Build history of the part. All positions in model axes, mm. Face numbers are marked on the shaded views. A direction names the side the tool comes from. Round coordinates to 2 decimals unless told otherwise and drop trailing zeros. Order: outer loops, then holes, each group sorted by start corner. A loop starts at its lowest first (then second) coordinate and runs counter-clockwise, first axis right, second up. Notation, with made-up numbers: M 16,39 L 61,39 A15 ccw 61,59 Z; hole C 4.5,52 d5. An arc over 180 degrees is marked long. One line per item, written item: value. Start each with the question number.
Item 1: Band-saw the part on A-A, the plane z = 7. Write the cut outline in (x, y).
Item 2: Probe L1, parallel to Z at x = 12.3, y = 0 (3 decimals); L2, parallel to Z at x = 14.55, y = 0; L3, parallel to X at y = -8, z = 7. List the from-to ranges inside material, lowest first.
Item 3: Tool access for the marked faces 1 and 2: list every direction of +Z, -Z, +X, -X, +Y, -Y with a clear straight run to the whole face (end or side of a thin tool).
Item 4: Band-saw the part on D-D, the plane x = 8.5. Write the cut outline in (y, z).
Item 5: Band-saw the part on B-B, the plane z = 17.75. Write the cut outline in (x, y) (3 decimals), then the cut area to 3 significant figures.
Item 6: Pin check, flat tips, straight feed: pin 1 (2.5 mm diameter, centred on y = -1.5, z = 17, fed in from +X); pin 2 (1 mm diameter, centred on x = -15, y = 10, fed in from -Z); pin 3 (4 mm diameter, centred on x = -7, z = 21, fed in from +Y). Stop position of each tip, or through.
Item 7: Two-plate mould, pull along X, no slides. Class the marked faces 3, 4 and 5: +X half, -X half, draft (parallel to the pull), parting line (faces both ways), or undercut.
```python
from build123d import *

# Parameters (mm, degrees)
SKETCH1_W               = 32
SKETCH1_H               = 27
BOSS_EXTRUDE1_DEPTH     = 35
FILLET1_R               = 2
CUT_EXTRUDE1_DEPTH      = 1
CUT_EXTRUDE1_DEPTH_BACK = 28
BOSS_EXTRUDE2_DEPTH     = 7
BOSS_EXTRUDE3_DEPTH     = 1.75
SKETCH5_W               = 2
SKETCH5_H               = 7
CUT_EXTRUDE2_DEPTH      = 33
CUT_EXTRUDE3_DEPTH      = 20
SKETCH7_W               = 2
SKETCH7_H               = 33
BOSS_EXTRUDE4_DEPTH     = 0.25
FILLET2_R               = 6
CUT_EXTRUDE5_DEPTH      = 4.5
SKETCH14_W              = 2.5
SKETCH14_H              = 20
CUT_EXTRUDE6_DEPTH      = 20
SKETCH16_W              = 2
SKETCH16_H              = 3.75
SKETCH16_H_2            = 2
BOSS_EXTRUDE5_DEPTH     = 20
BOSS_EXTRUDE6_DEPTH     = 20


with BuildPart() as part:
    # Sketch1 → Boss-Extrude1 (new body)
    with BuildSketch(Plane.XY):
        Rectangle(SKETCH1_W, SKETCH1_H)
    extrude(amount=BOSS_EXTRUDE1_DEPTH)

    # Fillet1
    fillet1_edges = [part.edges().sort_by_distance(p)[0] for p in [
        (16, -13.5, 17.5),
        (-16, -13.5, 17.5),
        (-16, 13.5, 17.5),
        (16, 13.5, 17.5),
    ]]
    fillet(fillet1_edges, radius=FILLET1_R)

    # Sketch2 → Cut-Extrude1 (cut, two sides)
    with BuildSketch(Plane.XZ.offset(13.5)) as cut_extrude1_sk:
        Polygon((-7.75, 0), (-7.75, 1.75), (-9.25, 1.75), (-9.25, 5.25), (9.25, 5.25), (9.25, 1.75), (7.75, 1.75), (7.75, 0), align=None)
    extrude(amount=CUT_EXTRUDE1_DEPTH, mode=Mode.SUBTRACT)
    extrude(cut_extrude1_sk.sketch, amount=-CUT_EXTRUDE1_DEPTH_BACK, mode=Mode.SUBTRACT)

    # Sketch3 → Boss-Extrude2 (add)
    with BuildSketch(Plane.XZ.offset(13.5)):
        Polygon((-7.75, 0), (-7.75, 1.75), (-9.25, 1.75), (-9.25, 5.25), (9.25, 5.25), (9.25, 1.75), (7.75, 1.75), (7.75, 0), align=None)
    extrude(amount=-BOSS_EXTRUDE2_DEPTH)

    # Sketch4 → Boss-Extrude3 (add)
    with BuildSketch(Plane(origin=(0, 0, 1.75), x_dir=(-1, 0, 0), z_dir=(0, 0, -1))):
        with BuildLine():
            Line((-7.75, 6.5), (-7.75, 5.5))
            ThreePointArc((-7.75, 5.5), (-7.5, 6), (-7.75, 6.5))
        make_face()
    boss_extrude3 = extrude(amount=BOSS_EXTRUDE3_DEPTH)

    # Mirror1: Boss-Extrude3 across plane
    add(boss_extrude3.mirror(Plane(origin=(0, 0, 0), x_dir=(0, 0, 1), z_dir=(1, 0, 0))))

    # Sketch5 → Cut-Extrude2 (cut)
    with BuildSketch(Plane(origin=(0, 0, 0), x_dir=(-1, 0, 0), z_dir=(0, 0, -1))):
        with Locations((0, -10)):
            Rectangle(SKETCH5_W, SKETCH5_H)
    extrude(amount=-CUT_EXTRUDE2_DEPTH, mode=Mode.SUBTRACT)

    # Sketch6 → Cut-Extrude3 (cut)
    with BuildSketch(Plane(origin=(0, 13.5, 0), x_dir=(1, 0, 0), z_dir=(0, 1, 0))):
        Polygon((-12.5, -7.75), (-12.5, -9.25), (-11.5, -9.25), (-11.5, -33), (11.5, -33), (11.5, -9.25), (12.5, -9.25), (12.5, -7.75), align=None)
    extrude(amount=-CUT_EXTRUDE3_DEPTH, mode=Mode.SUBTRACT)

    # Sketch7 → Boss-Extrude4 (add)
    with BuildSketch(Plane.XZ.offset(13.5)):
        with Locations((0, 16.5)):
            Rectangle(SKETCH7_W, SKETCH7_H)
    extrude(amount=-BOSS_EXTRUDE4_DEPTH)

    # Fillet2
    fillet2_edges = [part.edges().sort_by_distance(p)[0] for p in [
        (0, -13.25, 33),
    ]]
    fillet(fillet2_edges, radius=FILLET2_R)

    # Sketch9 → Cut-Revolve1 (revolve, cut)
    with BuildSketch(Plane(origin=(0, 0, 17.75), x_dir=(-1, 0, 0), z_dir=(0, 0, -1))):
        Polygon((-15, 4.25), (-14, 4.25), (-14, 3.325), (-11.5, 3.325), (-11.5, 0), (-16, 0), (-16, 3.75), (-15, 3.75), align=None)
    revolve(axis=Axis((16, 0, 17.75), (-1, 0, 0)), mode=Mode.SUBTRACT)

    # Sketch11 → Cut-Extrude5 (cut)
    with BuildSketch(Plane(origin=(-16, 0, 44), x_dir=(0, 0, -1), z_dir=(1, 0, 0))):
        with BuildLine():
            Line((24.25, 23), (24.25, 0))
            ThreePointArc((24.25, 0), (21, -3.25), (17.75, 0))
            Line((17.75, 0), (17.75, 23))
            ThreePointArc((17.75, 23), (21, 26.25), (24.25, 23))
        make_face()
    extrude(amount=CUT_EXTRUDE5_DEPTH, mode=Mode.SUBTRACT)

    # Sketch14 → Cut-Extrude6 (cut)
    with BuildSketch(Plane(origin=(0, 13.5, 0), x_dir=(1, 0, 0), z_dir=(0, 1, 0))):
        with Locations((-12.75, -23)):
            Rectangle(SKETCH14_W, SKETCH14_H)
    extrude(amount=-CUT_EXTRUDE6_DEPTH, mode=Mode.SUBTRACT)

    # Sketch16 → Boss-Extrude5 (add)
    with BuildSketch(Plane(origin=(0, 13.5, 0), x_dir=(1, 0, 0), z_dir=(0, 1, 0))):
        with Locations((-11, -13.125)):
            Rectangle(SKETCH16_W, SKETCH16_H)
        with Locations((-11, -32)):
            Rectangle(SKETCH16_W, SKETCH16_H_2)
    extrude(amount=-BOSS_EXTRUDE5_DEPTH)

    # Sketch20 → Boss-Extrude6 (add)
    with BuildSketch(Plane(origin=(0, 13.5, 0), x_dir=(1, 0, 0), z_dir=(0, 1, 0))):
        Polygon((-11.5, -9.25), (-10, -11.25), (-11.5, -11.25), align=None)
        Polygon((-10, -31), (-8.5, -33), (-10, -33), align=None)
    extrude(amount=-BOSS_EXTRUDE6_DEPTH)


solid = part.part
```
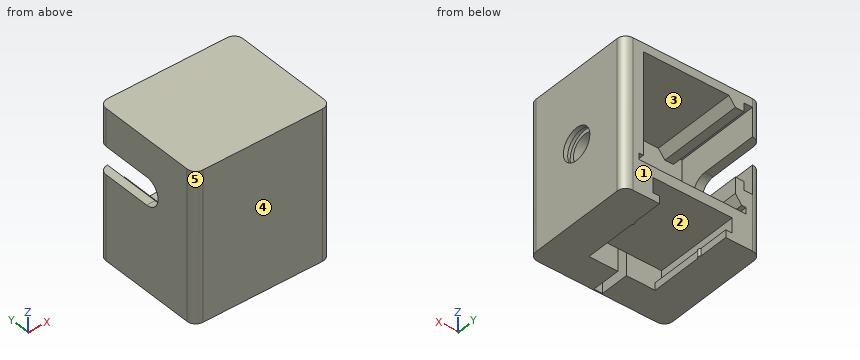
Output:
1. outline: M -16,-11.5 A2 ccw -14,-13.5 L 14,-13.5 A2 ccw 16,-11.5 L 16,11.5 A2 ccw 14,13.5 L -14,13.5 A2 ccw -16,11.5 Z; hole M -1,-13.25 L 1,-13.25 L 1,-6.5 L -1,-6.5 Z
2. L1: z = 0 to 7.75, 9.25 to 14.425, 21.075 to 35
2. L2: z = 0 to 13.5, 22 to 35
2. L3: x = -16 to -1, 1 to 16
3. face 1: +Z, -Z, +X, -X, +Y
3. face 2: +Y
4. outline: M -13.5,0 L 13.5,0 L 13.5,1.75 L -6.5,1.75 L -6.5,5.25 L 13.5,5.25 L 13.5,7.75 L -6.5,7.75 L -6.5,33 L 13.5,33 L 13.5,35 L -13.5,35 Z
5. outline: M -16,-11.5 A2 ccw -14,-13.5 L 14,-13.5 A2 ccw 16,-11.5 L 16,-3.75 L 15,-3.75 L 15,-4.25 L 14,-4.25 L 14,-3.325 L 11.5,-3.325 L 11.5,-6.5 L 1,-6.5 L 1,-13.25 L -1,-13.25 L -1,-6.5 L -14,-6.5 L -14,13.5 A2 ccw -16,11.5 Z; M 11.5,3.325 L 14,3.325 L 14,4.25 L 15,4.25 L 15,3.75 L 16,3.75 L 16,11.5 A2 ccw 14,13.5 L 11.5,13.5 Z
5. area: 304 mm²
6. pin 1: stops at x = -14
6. pin 2: stops at z = 0
6. pin 3: stops at y = -6.5
7. face 3: undercut
7. face 4: draft
7. face 5: -X half
